Build history of the part. All positions in model axes, mm. Give positions to 0.01 mm unless a question says otherwise; leave off trailing zeros. Order: outer loops, then holes, each group sorted by start corner. A loop starts at its lowest first (then second) coordinate and runs counter-clockwise, first axis right, second up. Notation, with made-up numbers: (9.25, 89) - (39.25, 89) arc R27 cw to (39.25, 113) - close; hole circle Ø8 at (56, -22). An arc over 180 degrees is marked (long way). Use a Markdown table: item, result. Add a question column.
(1) Mould opens along Y. For faces 1 (the face through (-19.85, 26.92, 1.52)), 2 (the face through (-1, -9, 3)) say: +Y half, -Y half, draft (parallel to the pull), parting line (faces both ways), or undercut.
(2) Slice it at D-D (y = 20). Write the cut outline in (x, z).
(3) Slice it at A-A (y = 0). Count the separate pieces of the cut face and the enclosed holes in it, then the cut area to 3 significant figures.
(4) Slice it at B-B (y = 42). Write the cut outline in (x, z), then the cut area to 3 significant figures.
(5) Wall check: line 1 (Y direction, x = -21, z = 2.3); line 2 (Y direction, x = -26.5, z = 2); line 3 (Y direction, x = -11, z = 1.45). Give the ranges that are in metal, low to high.
(6) Flat gauge pins, fed straight in: pin 1 (3.5 mm diameter, centred on x = 0, y = -12.5, fed in from +Z); pin 2 (1 mm diameter, centred on y = 13.5, z = 1, fed in from +X); pin 3 (0.8 mm diameter, centred on y = -35, z = 2, fed in from +X). Where does each tip first touch, or does it go through?
from build123d import *
from build123d.topology import SkipClean

# Parameters (mm, degrees)
EXTRUDE_1_OUTLINE_R      = 45
EXTRUDE_1_OUTLINE_R_2    = 2.1
EXTRUDE_1_OUTLINE_R_3    = 1.6
EXTRUDE_1_OUTLINE_R_4    = 1.3
EXTRUDE_1_OUTLINE_R_5    = 8
EXTRUDE_1_DEPTH          = 3
CUT_EXTRUDE_1_DEPTH      = 10
PATTERN_CIRCULAR_1_COUNT = 2
CUT_EXTRUDE_2_DEPTH      = 10
FILLET_1_R               = 2
CHAMFER_1_SIZE           = 1.5


# Read off the part's stored shape, not the designer's step: 凸台-拉伸1
with BuildPart() as part:
    # 凸台-拉伸1 outline → 凸台-拉伸1 (new body)
    with BuildSketch(Plane.XY):
        Circle(EXTRUDE_1_OUTLINE_R)
        with Locations((-29.69848481, -29.69848481)):
            Circle(EXTRUDE_1_OUTLINE_R_2, mode=Mode.SUBTRACT)
        with Locations((-17.320508076, -10)):
            Circle(EXTRUDE_1_OUTLINE_R_3, mode=Mode.SUBTRACT)
        with Locations((-10.825317547, -6.25)):
            Circle(EXTRUDE_1_OUTLINE_R_4, mode=Mode.SUBTRACT)
        with Locations((0, -42)):
            Circle(EXTRUDE_1_OUTLINE_R_2, mode=Mode.SUBTRACT)
        with Locations((29.69848481, -29.69848481)):
            Circle(EXTRUDE_1_OUTLINE_R_2, mode=Mode.SUBTRACT)
        with Locations((0, -20)):
            Circle(EXTRUDE_1_OUTLINE_R_3, mode=Mode.SUBTRACT)
        with Locations((0, -12.5)):
            Circle(EXTRUDE_1_OUTLINE_R_4, mode=Mode.SUBTRACT)
        with Locations((10.825317547, -6.25)):
            Circle(EXTRUDE_1_OUTLINE_R_4, mode=Mode.SUBTRACT)
        with Locations((17.320508076, -10)):
            Circle(EXTRUDE_1_OUTLINE_R_3, mode=Mode.SUBTRACT)
        with Locations((-42, 0)):
            Circle(EXTRUDE_1_OUTLINE_R_2, mode=Mode.SUBTRACT)
        with Locations((-17.320508076, 10)):
            Circle(EXTRUDE_1_OUTLINE_R_3, mode=Mode.SUBTRACT)
        with Locations((-10.825317547, 6.25)):
            Circle(EXTRUDE_1_OUTLINE_R_4, mode=Mode.SUBTRACT)
        with Locations((-29.69848481, 29.69848481)):
            Circle(EXTRUDE_1_OUTLINE_R_2, mode=Mode.SUBTRACT)
        Circle(EXTRUDE_1_OUTLINE_R_5, mode=Mode.SUBTRACT)
        with Locations((10.825317547, 6.25)):
            Circle(EXTRUDE_1_OUTLINE_R_4, mode=Mode.SUBTRACT)
        with Locations((17.320508076, 10)):
            Circle(EXTRUDE_1_OUTLINE_R_3, mode=Mode.SUBTRACT)
        with Locations((0, 12.5)):
            Circle(EXTRUDE_1_OUTLINE_R_4, mode=Mode.SUBTRACT)
        with Locations((0, 20)):
            Circle(EXTRUDE_1_OUTLINE_R_3, mode=Mode.SUBTRACT)
        with Locations((42, 0)):
            Circle(EXTRUDE_1_OUTLINE_R_2, mode=Mode.SUBTRACT)
        with Locations((0, 42)):
            Circle(EXTRUDE_1_OUTLINE_R_2, mode=Mode.SUBTRACT)
        with Locations((29.69848481, 29.69848481)):
            Circle(EXTRUDE_1_OUTLINE_R_2, mode=Mode.SUBTRACT)
    extrude(amount=EXTRUDE_1_DEPTH)

    # 草图2 → 切除-拉伸1 (cut)
    with BuildSketch(Plane.XY.offset(3)):
        with BuildLine():
            Line((4, 37.788887255), (4, 36.783148315))
            ThreePointArc((4, 36.783148315), (35.651970274, 9.896313233), (22.387428888, -29.4584967))
            Line((22.387428888, -29.4584967), (17.380966757, -24.452034569))
            ThreePointArc((17.380966757, -24.452034569), (16.963906124, -24.743198844), (16.541969004, -25.027250378))
            Line((16.541969004, -25.027250378), (22.290357636, -30.77563901))
            ThreePointArc((22.290357636, -30.77563901), (36.716063128, 9.794422308), (4, 37.788887255))
        make_face()
        with BuildLine():
            Line((-4, 37.788887255), (-4, 30.740852298))
            ThreePointArc((-4, 30.740852298), (26.614522572, 15.895508431), (25.168841559, -18.097773747))
            Line((25.168841559, -18.097773747), (24.452034569, -17.380966757))
            ThreePointArc((24.452034569, -17.380966757), (25.41530796, 15.93932625), (-5, 29.580398915))
            Line((-5, 29.580398915), (-5, 37.669616404))
            ThreePointArc((-5, 37.669616404), (-4.500395136, 37.732564763), (-4, 37.788887255))
        make_face()
    cut_extrude_1 = extrude(amount=-CUT_EXTRUDE_1_DEPTH, mode=Mode.SUBTRACT)

    # 阵列(圆周)1: 切除-拉伸1 ×2 about axis
    pattern_circular_1_axis = Axis((0, 0, 0), (0, 0, 1))
    for i in range(1, PATTERN_CIRCULAR_1_COUNT):
        add(cut_extrude_1.rotate(pattern_circular_1_axis, i * 360 / PATTERN_CIRCULAR_1_COUNT), mode=Mode.SUBTRACT)

    # 草图3 → 切除-拉伸2 (cut)
    with SkipClean():  # the faces are left unmerged after this step: merging them gives an invalid solid
        with BuildSketch(Plane.XY.offset(3)):
            with BuildLine():
                Line((-5, 37.669616404), (-5, 29.580398915))
                ThreePointArc((-5, 29.580398915), (-11.00894625, 27.907043958), (-16.541969004, 25.027250378))
                Line((-16.541969004, 25.027250378), (-22.290357636, 30.77563901))
                ThreePointArc((-22.290357636, 30.77563901), (-14.073828052, 35.297696298), (-5, 37.669616404))
            make_face()
            with BuildLine():
                Line((16.541969004, -25.027250378), (22.290357636, -30.77563901))
                ThreePointArc((22.290357636, -30.77563901), (14.073828052, -35.297696298), (5, -37.669616404))
                Line((5, -37.669616404), (5, -29.580398915))
                ThreePointArc((5, -29.580398915), (11.00894625, -27.907043958), (16.541969004, -25.027250378))
            make_face()
        extrude(amount=-CUT_EXTRUDE_2_DEPTH, mode=Mode.SUBTRACT)

    # 圆角1
    fillet_1_edges = [part.edges().sort_by_distance(p)[0] for p in [
        (-4, 37.788887255, 1.5),
        (-4, 30.740852298, 1.5),
        (17.380966757, -24.452034569, 1.5),
        (22.387428888, -29.4584967, 1.5),
        (4, -37.788887255, 1.5),
        (4, -30.740852298, 1.5),
        (-17.380966757, 24.452034569, 1.5),
        (-22.387428888, 29.4584967, 1.5),
    ]]
    fillet(fillet_1_edges, radius=FILLET_1_R)

    # 倒角1
    chamfer_1_edges = [part.edges().sort_by_distance(p)[0] for p in [
        (-1.3, 12.5, 3),
        (9.525317547, 6.25, 3),
        (9.525317547, -6.25, 3),
        (-1.3, -12.5, 3),
        (-12.125317547, -6.25, 3),
        (-12.125317547, 6.25, 3),
    ]]
    chamfer(chamfer_1_edges, length=CHAMFER_1_SIZE)


solid = part.part
Solution:
| question | item | result |
|---|---|---|
| 1 | face 1 | undercut |
| 1 | face 2 | draft |
| 2 | outline | (-40.31, 0) - (-32.31, 0) - (-32.31, 3) - (-40.31, 3) - close; (-31.13, 0) - (-1.6, 0) - (-1.6, 3) - (-31.13, 3) - close; (1.6, 0) - (22.36, 0) - (22.36, 3) - (1.6, 3) - close; (23.69, 0) - (31.13, 0) - (31.13, 3) - (23.69, 3) - close; (32.31, 0) - (40.31, 0) - (40.31, 3) - (32.31, 3) - close |
| 3 | separate pieces | 8 |
| 3 | enclosed holes | 0 |
| 3 | area | 185 mm2 |
| 4 | outline | (-16.16, 0) - (-2.1, 0) - (-2.1, 3) - (-16.16, 3) - close; (2.1, 0) - (16.16, 0) - (16.16, 3) - (2.1, 3) - close |
| 4 | area | 84.3 mm2 |
| 5 | line 1 | -39.8 to -31.67, -30.46 to -22.8, -21.42 to 28.07, 31.67 to 39.8 |
| 5 | line 2 | -36.37 to -27.24, -25.82 to -16.09, -14.06 to 14.06, 16.09 to 25.82, 27.24 to 36.37 |
| 5 | line 3 | -43.63 to -36.37, -35.33 to -28.98, -27.91 to -7.54, -4.96 to 4.96, 7.54 to 27.91, 36.37 to 43.63 |
| 6 | pin 1 | z = 1.95 |
| 6 | pin 2 | x = 43.08 |
| 6 | pin 3 | x = 28.77 |
